Geometry check sheet. Reference: the model listing, model coordinates, mm. A direction names the side the tool comes from. Give positions to 0.01 mm unless a question says otherwise; leave off trailing zeros. Order: outer loops, then holes, each group sorted by start corner. A loop starts at its lowest first (then second) coordinate and runs counter-clockwise, first axis right, second up. Notation, with made-up numbers: (58.25, 33.25) - (63.25, 33.25) arc R28 cw to (63.25, 52.25) - close; hole circle Ø7 at (56, 52.5). An arc over 180 degrees is marked (long way). Put each result on its own line as item: value. Start each with the question number.
```python
from build123d import *

# Parameters (mm, degrees)
SKETCH_1_W               = 39.05
SKETCH_1_H               = 35.07
SKETCH_1_R               = 1.65
SKETCH_1_R_2             = 1.25
EXTRUDE_1_DEPTH          = 3
EXTRUDE_2_DEPTH          = 1
EXTRUDE_2_DEPTH_BACK     = 9
SKETCH_2_W               = 5
SKETCH_2_H               = 35.07
CUT_EXTRUDE_3_DEPTH      = 41
CUT_EXTRUDE_3_DEPTH_BACK = 10
SKETCH_6_W               = 1
SKETCH_6_H               = 35.07
SKETCH_7_R               = 1.25
CUT_EXTRUDE_4_DEPTH      = 27
FILLET_6_R               = 3
FILLET_7_R               = 3
FILLET_8_R               = 3
SKETCH_13_R              = 2.76
CUT_EXTRUDE_7_DEPTH      = 3.2


with BuildPart() as part:
    # 草图1 → 凸台-拉伸1 (new body)
    with BuildSketch(Plane(origin=(0, 0, 0), x_dir=(-1, 0, 0), z_dir=(0, 0, 1))):
        with Locations((-56.669266884, 18.579160576)):
            Rectangle(SKETCH_1_W, SKETCH_1_H)
        with Locations(Location((-62.811349691, 23.836728616, 0), (0, 0, 180))):
            Circle(SKETCH_1_R, mode=Mode.SUBTRACT)
        with Locations(Location((-50.527184077, 13.321592536, 0), (0, 0, 180))):
            Circle(SKETCH_1_R, mode=Mode.SUBTRACT)
        with Locations(Location((-74.194266884, 25.614160576, 0), (0, 0, 180))):
            Circle(SKETCH_1_R_2, mode=Mode.SUBTRACT)
        with Locations(Location((-74.194266884, 11.544160576, 0), (0, 0, 180))):
            Circle(SKETCH_1_R_2, mode=Mode.SUBTRACT)
        with Locations(Location((-74.194266884, 18.579160576, 0), (0, 0, 180))):
            Circle(SKETCH_1_R_2, mode=Mode.SUBTRACT)
        with Locations(Location((-39.144266884, 25.614160576, 0), (0, 0, 180))):
            Circle(SKETCH_1_R_2, mode=Mode.SUBTRACT)
        with Locations(Location((-39.144266884, 18.579160576, 0), (0, 0, 180))):
            Circle(SKETCH_1_R_2, mode=Mode.SUBTRACT)
        with Locations(Location((-39.144266884, 11.544160576, 0), (0, 0, 180))):
            Circle(SKETCH_1_R_2, mode=Mode.SUBTRACT)
        with Locations(Location((-51.900012913, 22.58082967, 0), (0, 0, 180))):
            Circle(SKETCH_1_R, mode=Mode.SUBTRACT)
        with Locations(Location((-61.364857237, 14.469544513, 0), (0, 0, 180))):
            Circle(SKETCH_1_R, mode=Mode.SUBTRACT)
    extrude(amount=EXTRUDE_1_DEPTH)

    # 草图2 → 凸台-拉伸2 (add, two sides: drawn at the far end of the back side and taken through both)
    with BuildSketch(Plane(origin=(0, 0, 0), x_dir=(-1, 0, 0), z_dir=(0, 0, -1)).offset(-EXTRUDE_2_DEPTH_BACK)):
        with Locations((-73.694266884, -18.579160576)):
            Rectangle(SKETCH_2_W, SKETCH_2_H)
        with Locations((-39.644266884, -18.579160576)):
            Rectangle(SKETCH_2_W, SKETCH_2_H)
    extrude(amount=EXTRUDE_2_DEPTH + EXTRUDE_2_DEPTH_BACK)

    # 草图6 → 切除-拉伸3 (cut, two sides: drawn at the far end of the back side and taken through both)
    with BuildSketch(Plane(origin=(42.144266884, 0, 0), x_dir=(0, 0, -1), z_dir=(1, 0, 0)).offset(-CUT_EXTRUDE_3_DEPTH_BACK)):
        with Locations((0.5, -18.579160576)):
            Rectangle(SKETCH_6_W, SKETCH_6_H)
    extrude(amount=CUT_EXTRUDE_3_DEPTH + CUT_EXTRUDE_3_DEPTH_BACK, mode=Mode.SUBTRACT)

    # 草图7 → 切除-拉伸4 (cut)
    with BuildSketch(Plane(origin=(0, 0, 0), x_dir=(-1, 0, 0), z_dir=(0, 0, -1))):
        with Locations((-74.194266884, -11.544160576)):
            Circle(SKETCH_7_R)
        with Locations((-74.194266884, -18.579160576)):
            Circle(SKETCH_7_R)
        with Locations((-74.194266884, -25.614160576)):
            Circle(SKETCH_7_R)
        with Locations((-39.144266884, -11.544160576)):
            Circle(SKETCH_7_R)
        with Locations((-39.144266884, -18.579160576)):
            Circle(SKETCH_7_R)
        with Locations((-39.144266884, -25.614160576)):
            Circle(SKETCH_7_R)
    extrude(amount=-CUT_EXTRUDE_4_DEPTH, mode=Mode.SUBTRACT)

    # 圆角6
    fillet_6_edges = [part.edges().sort_by_distance(p)[0] for p in [
        (37.144266884, -36.114160576, 4.5),
    ]]
    fillet(fillet_6_edges, radius=FILLET_6_R)

    # 圆角7
    fillet_7_edges = [part.edges().sort_by_distance(p)[0] for p in [
        (37.144266884, -1.044160576, 4.5),
    ]]
    fillet(fillet_7_edges, radius=FILLET_7_R)

    # 圆角8
    fillet_8_edges = [part.edges().sort_by_distance(p)[0] for p in [
        (76.194266884, -1.044160576, 4.5),
        (76.194266884, -36.114160576, 4.5),
    ]]
    fillet(fillet_8_edges, radius=FILLET_8_R)

    # 草图13 → 切除-拉伸7 (cut)
    with BuildSketch(Plane(origin=(0, 0, 0), x_dir=(-1, 0, 0), z_dir=(0, 0, -1))):
        with Locations((-74.194266884, -11.544160576)):
            Circle(SKETCH_13_R)
        with Locations((-74.194266884, -18.579160576)):
            Circle(SKETCH_13_R)
        with Locations((-74.194266884, -25.614160576)):
            Circle(SKETCH_13_R)
        with Locations((-39.144266884, -11.544160576)):
            Circle(SKETCH_13_R)
        with Locations((-39.144266884, -18.579160576)):
            Circle(SKETCH_13_R)
        with Locations((-39.144266884, -25.614160576)):
            Circle(SKETCH_13_R)
    extrude(amount=-CUT_EXTRUDE_7_DEPTH, mode=Mode.SUBTRACT)


solid = part.part
```
Item 1: Cross-section at B-B (x = 63.5). Enter the section's corners in (y, z), and give its area (3 significant figures).
Item 2: Cross-section at C-C (y = -30). Enter the section's corners in (x, z), and give its area (3 significant figures).
Item 3: Set-up check for faces 4 (the face through (51.414, -11.93, 1.479)), 5 (the face through (71.436, -25.706, 1.578)), 6 (the face through (71.194, -19, 6)): record each of +Z, -Z, +X, -X, +Y, -Y from which the full face is reachable in a straight line by a thin tool's end or side.
Item 4: Cross-section at A-A (z = 3.75). Enter the section's corners in (x, y), and give its area (3 significant figures).
Item 5: Gauge pin test, flat ends, axial feed: pin 1 Ø4 at (x, y) = (63.5, -22.5) entering from -Z; pin 2 Ø5 at (x, y) = (74.19, -25.61) entering from -Z. Record the tip position at first contact, or that the pin passes through.
Item 6: Thickness scan on line 1 along X through (y, z) = (-32.5, 4.5); line 2 along X through (y, z) = (-11, 6); line 3 along Z through (x, y) = (50.5, -20.5). Record the ranges inside material, lowest first.
Item 7: Release check for a two-part mould opening along X. For faces 1 (the face through (60.6, -36.114, 2.6)), 2 (the face through (76.194, -19, 5)), 3 (the face through (75.443, -11.489, 6.059)) record: +X half, -X half, draft (parallel to the pull), parting line (faces both ways), or undercut.
Item 8: Cross-section at D-D (z = 0.5). Enter the section's corners in (x, y).
Recorded:
1. outline: (-36.11, 0) - (-25.34, 0) - (-25.34, 3) - (-36.11, 3) - close; (-22.34, 0) - (-1.04, 0) - (-1.04, 3) - (-22.34, 3) - close
1. area: 96.2 mm^2
2. outline: (37.14, 0) - (76.19, 0) - (76.19, 9) - (71.19, 9) - (71.19, 3) - (42.14, 3) - (42.14, 9) - (37.14, 9) - close
2. area: 177 mm^2
3. face 4: +Z, -Z
3. face 5: -Z
3. face 6: +Z, +Y, -Y
4. outline: (37.14, -33.11) arc R3 ccw to (40.14, -36.11) - (42.14, -36.11) - (42.14, -1.04) - (40.14, -1.04) arc R3 ccw to (37.14, -4.04) - close; (71.19, -36.11) - (73.19, -36.11) arc R3 ccw to (76.19, -33.11) - (76.19, -4.04) arc R3 ccw to (73.19, -1.04) - (71.19, -1.04) - close; hole circle Ø2.5 at (39.14, -25.61); hole circle Ø2.5 at (39.14, -18.58); hole circle Ø2.5 at (39.14, -11.54); hole circle Ø2.5 at (74.19, -25.61); hole circle Ø2.5 at (74.19, -18.58); hole circle Ø2.5 at (74.19, -11.54)
4. area: 314 mm^2
5. pin 1: stops at z = 0
5. pin 2: stops at z = 3.2
6. line 1: x = 37.14 to 42.14, 71.19 to 76.19
6. line 2: x = 37.14 to 38.02, 40.27 to 42.14, 71.19 to 73.07, 75.32 to 76.19
6. line 3: z = 0 to 3
7. face 1: draft
7. face 2: +X half
7. face 3: undercut
8. outline: (37.14, -33.11) arc R3 ccw to (40.14, -36.11) - (73.19, -36.11) arc R3 ccw to (76.19, -33.11) - (76.19, -27.52) arc R2.76 cw (long way) to (76.19, -23.71) - (76.19, -20.48) arc R2.76 cw (long way) to (76.19, -16.68) - (76.19, -13.45) arc R2.76 cw (long way) to (76.19, -9.64) - (76.19, -4.04) arc R3 ccw to (73.19, -1.04) - (40.14, -1.04) arc R3 ccw to (37.14, -4.04) - (37.14, -9.64) arc R2.76 cw (long way) to (37.14, -13.45) - (37.14, -16.68) arc R2.76 cw (long way) to (37.14, -20.48) - (37.14, -23.71) arc R2.76 cw (long way) to (37.14, -27.52) - close; hole circle Ø3.3 at (50.53, -13.32); hole circle Ø3.3 at (51.9, -22.58); hole circle Ø3.3 at (61.36, -14.47); hole circle Ø3.3 at (62.81, -23.84)
